from build123d import *

# Parameters (mm, degrees)
F0_R     = 74.446601
F1_DEPTH = 25.4
F2_R     = 58.130128
F3_DEPTH = 66.04
F5_DEPTH = 67.564
F6_R     = 33.669878
F7_DEPTH = 55.626


with BuildPart() as f1:
    # F0 (on Front) → F1 (new body)
    with BuildSketch(Plane.XZ):
        Circle(F0_R)
    extrude(amount=F1_DEPTH)

    # F2 (on face) → F3 (join)
    with BuildSketch(Plane(origin=(0, 0, 0), x_dir=(-1, 0, 0), z_dir=(0, 1, 0))):
        Circle(F2_R)
    extrude(amount=F3_DEPTH)

    # F4 (on face) → F5 (cut)
    with BuildSketch(Plane(origin=(0, 66.04, 0), x_dir=(-1, 0, 0), z_dir=(0, 1, 0))):
        Polygon((24.31692, -48.409281), (54.082127, -3.14557), (29.765207, 45.263711), (-24.31692, 48.409281), (-54.082127, 3.14557), (-29.765207, -45.263711), align=None)
    extrude(amount=-F5_DEPTH, mode=Mode.SUBTRACT)

    # F6 (on face) → F7 (join)
    with BuildSketch(Plane.XZ.offset(25.4)):
        Circle(F6_R)
    extrude(amount=F7_DEPTH)

    # F8: F1 across face


with BuildPart() as f1_1:
    add(f1.part)
    add(f1.part.mirror(Plane.XZ.offset(81.026)))


solid = f1_1.part
CAD build for the part. Positions are in the model's coordinates, mm. A direction names the side the tool comes from. Round coordinates to 2 decimals unless told otherwise and drop trailing zeros. Order: outer loops, then holes, each group sorted by start corner. A loop starts at its lowest first (then second) coordinate and runs counter-clockwise, first axis right, second up. Notation, with made-up numbers: (-34.75, -33.5) -> (20.25, -33.5) arc R19 cw to (20.25, 3.5) -> close; hole circle Ø8 at (37, 11.25). An arc over 180 degrees is marked (long way). Write each question's results on one line, items separated by ' | '.
1. Pull direction X, two halves, no side cores. Call faces 1 (the face through (42.84, 32.56, 39.29)), 2 (the face through (5, 66.04, -47)), 3 (the face through (-3.103, -194.783, 46.814)): pulls with the +X half, pulls with the -X half, needs draft (parallel to the pull), parting line crosses it, or undercut.
Findings below:
face 1: parting line crosses it | face 2: needs draft | face 3: undercut
2. Cut at C-C (x = -39.5). Give the cut face in (y, z).
Findings below:
outline: (-228.09, -42.65) -> (-162.05, -42.65) -> (-162.05, -63.1) -> (-136.65, -63.1) -> (-136.65, 63.1) -> (-162.05, 63.1) -> (-162.05, 42.65) -> (-228.09, 42.65) -> (-228.09, 25.88) -> (-160.53, 25.88) -> (-160.53, -25.32) -> (-228.09, -25.32) -> close; (-25.4, -63.1) -> (0, -63.1) -> (0, -42.65) -> (66.04, -42.65) -> (66.04, -25.32) -> (-1.52, -25.32) -> (-1.52, 25.88) -> (66.04, 25.88) -> (66.04, 42.65) -> (0, 42.65) -> (0, 63.1) -> (-25.4, 63.1) -> close
3. Wall check: line 1 along Y through (x, z) = (14.5, -63.5); line 2 along Y through (x, z) = (-32, 29.5); line 3 along Y through (x, z) = (21, -12). Give the ranges that are in metal, low to high. Write a range as [from, to].
Findings below:
line 1: y = [-162.05, -136.65], [-25.4, 0] | line 2: y = [-160.53, -136.65], [-25.4, -1.52] | line 3: y = [-160.53, -1.52]
4. 3-axis set-ups, long thin cutter, end or side, ignore diameter. For faces 4 (the face through (32, -25.4, -16)), 5 (the face through (42.84, -194.61, 39.29)), 6 (the face through (-16.139, -149.53, -72.676)), 7 (the face through (-38.991, 32.731, -26.094)): which of +Z, -Z, +X, -X, +Y, -Y reach the whole face in a straight line?
Findings below:
face 4: none | face 5: -Y | face 6: +Y, -Y | face 7: +Y
5. Cut at B-B (z = 54). Give the cut face in (x, y), plus the area to 3 significant figures.
Findings below:
outline: (-51.25, -162.05) -> (-21.52, -162.05) -> (-21.52, -228.09) -> (21.52, -228.09) -> (21.52, -162.05) -> (51.25, -162.05) -> (51.25, -136.65) -> (-51.25, -136.65) -> close; (-51.25, -25.4) -> (51.25, -25.4) -> (51.25, 0) -> (21.52, 0) -> (21.52, 66.04) -> (-21.52, 66.04) -> (-21.52, 0) -> (-51.25, 0) -> close | area: 10,900 mm²
6. Flat gauge pins, fed straight in: P1, Ø1.5, axis at y = 32, z = -32.5, coming from the -X side; P2, Ø10, axis at x = 48, z = -53.5, coming from the +Y side; P3, Ø8, axis at y = -75.5, z = -10, coming from the -X side. Where does each tip first touch, or does it go through?
Findings below:
P1: stops at x = -48.69 | P2: stops at y = 0 | P3: stops at x = -33.13
7. Cut at D-D (x = -3). Give the cut face in (y, z).
Findings below:
outline: (-228.09, -58.05) -> (-162.05, -58.05) -> (-162.05, -74.39) -> (-136.65, -74.39) -> (-136.65, -33.54) -> (-25.4, -33.54) -> (-25.4, -74.39) -> (0, -74.39) -> (0, -58.05) -> (66.04, -58.05) -> (66.04, -47.17) -> (-1.52, -47.17) -> (-1.52, 46.82) -> (66.04, 46.82) -> (66.04, 58.05) -> (0, 58.05) -> (0, 74.39) -> (-25.4, 74.39) -> (-25.4, 33.54) -> (-136.65, 33.54) -> (-136.65, 74.39) -> (-162.05, 74.39) -> (-162.05, 58.05) -> (-228.09, 58.05) -> (-228.09, 46.82) -> (-160.53, 46.82) -> (-160.53, -47.17) -> (-228.09, -47.17) -> close
8. Cut at A-A (y = -169). Give the cut face in (x, z).
Findings below:
outline: circle Ø116.26 at (0, 0); hole (-54.08, -3.15) -> (-24.32, -48.41) -> (29.77, -45.26) -> (54.08, 3.15) -> (24.32, 48.41) -> (-29.77, 45.26) -> close
